Source: CAD feature listing. Evaluate the final solid. Frame: model axes, mm. Face numbers are marked on the shaded views. A direction names the side the tool comes from. Round coordinates to 2 decimals unless told otherwise and drop trailing zeros. Loops run counter-clockwise (first coordinate to the right, second up) from the corner with the lowest first, then second, coordinate; pieces in that order, holes last. Notation, with made-up numbers: (-26.5, -35.5) -> (10.5, -35.5) arc R31 ccw to (10.5, -0.5) -> close; hole circle Ø9 at (-23, 31.5). An arc over 180 degrees is marked (long way). Put each result on its own line as item: value. Start each with the question number.
1. Draft query along X for the marked faces 3, 4 and 5. Return one class per face: pulls with the +X half, pulls with the -X half, needs draft (parallel to the pull), parting line crosses it, or undercut.
2. Contact query for a flat-ended pin moving along its axis: pin 1 (3 mm diameter, centred on x = -38, z = 46, fed in from +Y). Output: stop coordinate, or through.
3. Cut plane C-C (x = -69). Return the cut outline in (y, z), then the cut area to 3 significant figures.
4. Cut plane B-B (z = 25.5). Return the cut outline in (x, y).
5. Set-up query: the marked faces 1 and 2. Return all of +Z, -Z, +X, -X, +Y, -Y with unobstructed straight access to the full face (end or side cutting, diameter ignored); none if empty.
6. Material intervals for L1, parallel to Z at x = -6.5, y = 14.5; L2, parallel to X at y = 52, z = -3; L3, parallel to Y at x = -57, z = 78, sorted ascending.
7. Cut plane A-A (y = 41). Return the cut outline in (x, z), then the cut area to 3 significant figures.
```python
from build123d import *

# Parameters (mm, degrees)
BOSS_EXTRUDE1_DEPTH = 80
SKETCH2_R           = 4.778019897
BOSS_EXTRUDE4_DEPTH = 3


with BuildPart() as part:
    # Sketch1 → Boss-Extrude1 (new body)
    with BuildSketch(Plane(origin=(0, 0, 0), x_dir=(1, 0, 0), z_dir=(0, 1, 0))):
        with BuildLine():
            ThreePointArc((-83.878172589, 11.35786802), (-80.949240401, 18.428935832), (-73.878172589, 21.35786802))
            Line((-73.878172589, 21.35786802), (12.121827411, 21.35786802))
            ThreePointArc((12.121827411, 21.35786802), (19.192895223, 18.428935832), (22.121827411, 11.35786802))
            Line((22.121827411, 11.35786802), (22.121827411, -74.64213198))
            ThreePointArc((22.121827411, -74.64213198), (19.192895223, -81.713199792), (12.121827411, -84.64213198))
            Line((12.121827411, -84.64213198), (-73.878172589, -84.64213198))
            ThreePointArc((-73.878172589, -84.64213198), (-80.949240401, -81.713199792), (-83.878172589, -74.64213198))
            Line((-83.878172589, -74.64213198), (-83.878172589, 11.35786802))
        make_face()
        with BuildLine():
            Line((-70.878172589, 18.35786802), (9.121827411, 18.35786802))
            ThreePointArc((9.121827411, 18.35786802), (16.192895223, 15.428935832), (19.121827411, 8.35786802))
            Line((19.121827411, 8.35786802), (19.121827411, -71.64213198))
            ThreePointArc((19.121827411, -71.64213198), (16.192895223, -78.713199792), (9.121827411, -81.64213198))
            Line((9.121827411, -81.64213198), (-70.878172589, -81.64213198))
            ThreePointArc((-70.878172589, -81.64213198), (-77.949240401, -78.713199792), (-80.878172589, -71.64213198))
            Line((-80.878172589, -71.64213198), (-80.878172589, 8.35786802))
            ThreePointArc((-80.878172589, 8.35786802), (-77.949240401, 15.428935832), (-70.878172589, 18.35786802))
        make_face(mode=Mode.SUBTRACT)
    extrude(amount=BOSS_EXTRUDE1_DEPTH)

    # Sketch2 → Boss-Extrude4 (add)
    with BuildSketch(Plane.XZ):
        with BuildLine():
            Line((-83.878172589, 74.64213198), (-83.878172589, -11.35786802))
            ThreePointArc((-83.878172589, -11.35786802), (-80.949240401, -18.428935832), (-73.878172589, -21.35786802))
            Line((-73.878172589, -21.35786802), (12.121827411, -21.35786802))
            ThreePointArc((12.121827411, -21.35786802), (19.192895223, -18.428935832), (22.121827411, -11.35786802))
            Line((22.121827411, -11.35786802), (22.121827411, 74.64213198))
            ThreePointArc((22.121827411, 74.64213198), (19.192895223, 81.713199792), (12.121827411, 84.64213198))
            Line((12.121827411, 84.64213198), (-73.878172589, 84.64213198))
            ThreePointArc((-73.878172589, 84.64213198), (-80.949240401, 81.713199792), (-83.878172589, 74.64213198))
        make_face()
        with BuildLine():
            ThreePointArc((19.121827411, -8.35786802), (16.192895223, -15.428935832), (9.121827411, -18.35786802))
            Line((9.121827411, -18.35786802), (-70.878172589, -18.35786802))
            ThreePointArc((-70.878172589, -18.35786802), (-77.949240401, -15.428935832), (-80.878172589, -8.35786802))
            Line((-80.878172589, -8.35786802), (-80.878172589, 71.64213198))
            ThreePointArc((-80.878172589, 71.64213198), (-77.949240401, 78.713199792), (-70.878172589, 81.64213198))
            Line((-70.878172589, 81.64213198), (9.121827411, 81.64213198))
            ThreePointArc((9.121827411, 81.64213198), (16.192895223, 78.713199792), (19.121827411, 71.64213198))
            Line((19.121827411, 71.64213198), (19.121827411, -8.35786802))
        make_face(mode=Mode.SUBTRACT)
        with BuildLine():
            Line((9.121827411, -18.35786802), (-70.878172589, -18.35786802))
            ThreePointArc((-70.878172589, -18.35786802), (-77.949240401, -15.428935832), (-80.878172589, -8.35786802))
            Line((-80.878172589, -8.35786802), (-80.878172589, 71.64213198))
            ThreePointArc((-80.878172589, 71.64213198), (-77.949240401, 78.713199792), (-70.878172589, 81.64213198))
            Line((-70.878172589, 81.64213198), (9.121827411, 81.64213198))
            ThreePointArc((9.121827411, 81.64213198), (16.192895223, 78.713199792), (19.121827411, 71.64213198))
            Line((19.121827411, 71.64213198), (19.121827411, -8.35786802))
            ThreePointArc((19.121827411, -8.35786802), (16.192895223, -15.428935832), (9.121827411, -18.35786802))
        make_face()
        with Locations(Location((13.968668107, -4.778019897, 0), (0, 0, 270))):
            Circle(SKETCH2_R, mode=Mode.SUBTRACT)
    extrude(amount=BOSS_EXTRUDE4_DEPTH)


solid = part.part
```
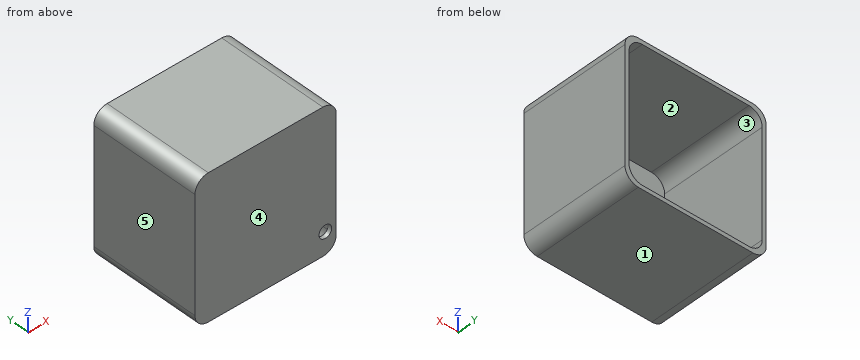
Solution:
1. face 3: undercut
1. face 4: needs draft
1. face 5: pulls with the -X half
2. pin 1: stops at y = 0
3. outline: (-3, -21.36) -> (80, -21.36) -> (80, -18.36) -> (0, -18.36) -> (0, 81.64) -> (80, 81.64) -> (80, 84.64) -> (-3, 84.64) -> close
3. area: 798 mm^2
4. outline: (-83.88, -3) -> (22.12, -3) -> (22.12, 80) -> (19.12, 80) -> (19.12, 0) -> (-80.88, 0) -> (-80.88, 80) -> (-83.88, 80) -> close
5. face 1: -Z, +X, -X, +Y, -Y
5. face 2: +Y
6. L1: z = -21.36 to -18.36, 81.64 to 84.64
6. L2: x = -83.88 to -80.88, 19.12 to 22.12
6. L3: y = -3 to 0
7. outline: (-83.88, -11.36) arc R10 ccw to (-73.88, -21.36) -> (12.12, -21.36) arc R10 ccw to (22.12, -11.36) -> (22.12, 74.64) arc R10 ccw to (12.12, 84.64) -> (-73.88, 84.64) arc R10 ccw to (-83.88, 74.64) -> close; hole (-80.88, -8.36) arc R10 ccw to (-70.88, -18.36) -> (9.12, -18.36) arc R10 ccw to (19.12, -8.36) -> (19.12, 71.64) arc R10 ccw to (9.12, 81.64) -> (-70.88, 81.64) arc R10 ccw to (-80.88, 71.64) -> close
7. area: 1,240 mm^2
